```python
from build123d import *

# Parameters (mm, degrees)
F1_DEPTH = 0.25


with BuildPart() as f1:
    # F0 (on Top) → F1 (new body)
    with BuildSketch(Plane.XY):
        with BuildLine():
            ThreePointArc((-0.5, -73.9983107915), (-52.3259018078, -52.3259018078), (-73.9983107915, -0.5))
            Line((-73.9983107915, -0.5), (-49.9974999375, -0.5))
            Line((-49.9974999375, -0.5), (-48.9974489132, -0.5))
            ThreePointArc((-48.9974489132, -0.5), (-49, 0), (-48.9974489132, 0.5))
            ThreePointArc((-48.9974489132, 0.5), (-34.6482322781, 34.6482322781), (-0.5, 48.9974489132))
            Line((-0.5, 48.9974489132), (-0.5, 49.9974999375))
            ThreePointArc((-0.5, 49.9974999375), (-35.3553390593, 35.3553390593), (-49.9974999375, 0.5))
            Line((-49.9974999375, 0.5), (-73.9983107915, 0.5))
            ThreePointArc((-73.9983107915, 0.5), (-52.3259018078, 52.3259018078), (-0.5, 73.9983107915))
            Line((-0.5, 73.9983107915), (-0.5, 74.9983333148))
            ThreePointArc((-0.5, 74.9983333148), (-53.033008589, 53.033008589), (-74.9983333148, 0.5))
            Line((-74.9983333148, 0.5), (-74.9983333148, -0.5))
            ThreePointArc((-74.9983333148, -0.5), (-53.033008589, -53.033008589), (-0.5, -74.9983333148))
            Line((-0.5, -74.9983333148), (-0.5, -73.9983107915))
        make_face()
        with BuildLine():
            Line((-0.5, -49.9974999375), (-0.5, -73.9983107915))
            ThreePointArc((-0.5, -73.9983107915), (0, -74), (0.5, -73.9983107915))
            Line((0.5, -73.9983107915), (0.5, -49.9974999375))
            ThreePointArc((0.5, -49.9974999375), (0, -50), (-0.5, -49.9974999375))
        make_face()
        with BuildLine():
            ThreePointArc((0.5, -73.9983107915), (0, -74), (-0.5, -73.9983107915))
            Line((-0.5, -73.9983107915), (-0.5, -74.9983333148))
            Line((-0.5, -74.9983333148), (0.5, -74.9983333148))
            Line((0.5, -74.9983333148), (0.5, -73.9983107915))
        make_face()
        with BuildLine():
            Line((-48.9974489132, -0.5), (-49.9974999375, -0.5))
            ThreePointArc((-49.9974999375, -0.5), (-35.3553390593, -35.3553390593), (-0.5, -49.9974999375))
            ThreePointArc((-0.5, -49.9974999375), (0, -50), (0.5, -49.9974999375))
            Line((0.5, -49.9974999375), (0.5, -48.9974489132))
            ThreePointArc((0.5, -48.9974489132), (0, -49), (-0.5, -48.9974489132))
            ThreePointArc((-0.5, -48.9974489132), (-34.6482322781, -34.6482322781), (-48.9974489132, -0.5))
        make_face()
        with BuildLine():
            ThreePointArc((73.9983107915, -0.5), (52.3259018078, -52.3259018078), (0.5, -73.9983107915))
            Line((0.5, -73.9983107915), (0.5, -74.9983333148))
            ThreePointArc((0.5, -74.9983333148), (53.033008589, -53.033008589), (74.9983333148, -0.5))
            Line((74.9983333148, -0.5), (73.9983107915, -0.5))
        make_face()
        with BuildLine():
            ThreePointArc((-48.9974489132, 0.5), (-49, 0), (-48.9974489132, -0.5))
            Line((-48.9974489132, -0.5), (-24.9949994999, -0.5))
            Line((-24.9949994999, -0.5), (-23.9947911014, -0.5))
            ThreePointArc((-23.9947911014, -0.5), (-24, 0), (-23.9947911014, 0.5))
            ThreePointArc((-23.9947911014, 0.5), (-16.9705627485, 16.9705627485), (-0.5, 23.9947911014))
            Line((-0.5, 23.9947911014), (-0.5, 24.9949994999))
            ThreePointArc((-0.5, 24.9949994999), (-17.6776695297, 17.6776695297), (-24.9949994999, 0.5))
            Line((-24.9949994999, 0.5), (-48.9974489132, 0.5))
        make_face()
        with BuildLine():
            Line((49.9974999375, -0.5), (73.9983107915, -0.5))
            ThreePointArc((73.9983107915, -0.5), (74, 0), (73.9983107915, 0.5))
            Line((73.9983107915, 0.5), (49.9974999375, 0.5))
            ThreePointArc((49.9974999375, 0.5), (50, 0), (49.9974999375, -0.5))
        make_face()
        with BuildLine():
            ThreePointArc((73.9983107915, 0.5), (74, 0), (73.9983107915, -0.5))
            Line((73.9983107915, -0.5), (74.9983333148, -0.5))
            Line((74.9983333148, -0.5), (74.9983333148, 0.5))
            Line((74.9983333148, 0.5), (73.9983107915, 0.5))
        make_face()
        with BuildLine():
            Line((0.5, -48.9974489132), (0.5, -49.9974999375))
            ThreePointArc((0.5, -49.9974999375), (35.3553390593, -35.3553390593), (49.9974999375, -0.5))
            Line((49.9974999375, -0.5), (48.9974489132, -0.5))
            ThreePointArc((48.9974489132, -0.5), (34.6482322781, -34.6482322781), (0.5, -48.9974489132))
        make_face()
        with BuildLine():
            ThreePointArc((-74.9983333148, 0.5), (-75, 0), (-74.9983333148, -0.5))
            Line((-74.9983333148, -0.5), (-74.9983333148, 0.5))
        make_face()
        with BuildLine():
            Line((-23.9947911014, -0.5), (-24.9949994999, -0.5))
            ThreePointArc((-24.9949994999, -0.5), (-17.6776695297, -17.6776695297), (-0.5, -24.9949994999))
            Line((-0.5, -24.9949994999), (-0.5, -48.9974489132))
            ThreePointArc((-0.5, -48.9974489132), (0, -49), (0.5, -48.9974489132))
            Line((0.5, -48.9974489132), (0.5, -24.9949994999))
            Line((0.5, -24.9949994999), (0.5, -23.9947911014))
            Line((0.5, -23.9947911014), (0.5, -2.4494897428))
            Line((0.5, -2.4494897428), (0.5, -0.5))
            Line((0.5, -0.5), (2.4494897428, -0.5))
            Line((2.4494897428, -0.5), (23.9947911014, -0.5))
            Line((23.9947911014, -0.5), (24.9949994999, -0.5))
            ThreePointArc((24.9949994999, -0.5), (25, 0), (24.9949994999, 0.5))
            Line((24.9949994999, 0.5), (23.9947911014, 0.5))
            Line((23.9947911014, 0.5), (2.4494897428, 0.5))
            Line((2.4494897428, 0.5), (0.5, 0.5))
            Line((0.5, 0.5), (-0.5, 0.5))
            Line((-0.5, 0.5), (-0.5, -0.5))
            Line((-0.5, -0.5), (-0.5, -2.4494897428))
            Line((-0.5, -2.4494897428), (-0.5, -23.9947911014))
            ThreePointArc((-0.5, -23.9947911014), (-16.9705627485, -16.9705627485), (-23.9947911014, -0.5))
        make_face()
        with BuildLine():
            ThreePointArc((0.5, 73.9983107915), (52.3259018078, 52.3259018078), (73.9983107915, 0.5))
            Line((73.9983107915, 0.5), (74.9983333148, 0.5))
            ThreePointArc((74.9983333148, 0.5), (53.033008589, 53.033008589), (0.5, 74.9983333148))
            Line((0.5, 74.9983333148), (0.5, 73.9983107915))
        make_face()
        with BuildLine():
            Line((48.9974489132, -0.5), (49.9974999375, -0.5))
            ThreePointArc((49.9974999375, -0.5), (50, 0), (49.9974999375, 0.5))
            Line((49.9974999375, 0.5), (48.9974489132, 0.5))
            ThreePointArc((48.9974489132, 0.5), (49, 0), (48.9974489132, -0.5))
        make_face()
        with BuildLine():
            Line((-0.5, 49.9974999375), (-0.5, 48.9974489132))
            ThreePointArc((-0.5, 48.9974489132), (0, 49), (0.5, 48.9974489132))
            Line((0.5, 48.9974489132), (0.5, 49.9974999375))
            ThreePointArc((0.5, 49.9974999375), (0, 50), (-0.5, 49.9974999375))
        make_face()
        with BuildLine():
            ThreePointArc((0.5, 48.9974489132), (0, 49), (-0.5, 48.9974489132))
            Line((-0.5, 48.9974489132), (-0.5, 24.9949994999))
            Line((-0.5, 24.9949994999), (-0.5, 23.9947911014))
            ThreePointArc((-0.5, 23.9947911014), (0, 24), (0.5, 23.9947911014))
            ThreePointArc((0.5, 23.9947911014), (16.9705627485, 16.9705627485), (23.9947911014, 0.5))
            Line((23.9947911014, 0.5), (24.9949994999, 0.5))
            ThreePointArc((24.9949994999, 0.5), (17.6776695297, 17.6776695297), (0.5, 24.9949994999))
            Line((0.5, 24.9949994999), (0.5, 48.9974489132))
        make_face()
        with BuildLine():
            ThreePointArc((-23.9947911014, 0.5), (-24, 0), (-23.9947911014, -0.5))
            Line((-23.9947911014, -0.5), (-2.4494897428, -0.5))
            Line((-2.4494897428, -0.5), (-0.5, -0.5))
            Line((-0.5, -0.5), (-0.5, 0.5))
            Line((-0.5, 0.5), (-2.4494897428, 0.5))
            Line((-2.4494897428, 0.5), (-23.9947911014, 0.5))
        make_face()
        with BuildLine():
            Line((0.5, 49.9974999375), (0.5, 73.9983107915))
            ThreePointArc((0.5, 73.9983107915), (0, 74), (-0.5, 73.9983107915))
            Line((-0.5, 73.9983107915), (-0.5, 49.9974999375))
            ThreePointArc((-0.5, 49.9974999375), (0, 50), (0.5, 49.9974999375))
        make_face()
        with BuildLine():
            ThreePointArc((-0.5, 73.9983107915), (0, 74), (0.5, 73.9983107915))
            Line((0.5, 73.9983107915), (0.5, 74.9983333148))
            Line((0.5, 74.9983333148), (-0.5, 74.9983333148))
            Line((-0.5, 74.9983333148), (-0.5, 73.9983107915))
        make_face()
        with BuildLine():
            Line((48.9974489132, 0.5), (49.9974999375, 0.5))
            ThreePointArc((49.9974999375, 0.5), (35.3553390593, 35.3553390593), (0.5, 49.9974999375))
            Line((0.5, 49.9974999375), (0.5, 48.9974489132))
            ThreePointArc((0.5, 48.9974489132), (34.6482322781, 34.6482322781), (48.9974489132, 0.5))
        make_face()
        with BuildLine():
            Line((24.9949994999, -0.5), (48.9974489132, -0.5))
            ThreePointArc((48.9974489132, -0.5), (49, 0), (48.9974489132, 0.5))
            Line((48.9974489132, 0.5), (24.9949994999, 0.5))
            ThreePointArc((24.9949994999, 0.5), (25, 0), (24.9949994999, -0.5))
        make_face()
        with BuildLine():
            Line((0.5, -23.9947911014), (0.5, -24.9949994999))
            ThreePointArc((0.5, -24.9949994999), (17.6776695297, -17.6776695297), (24.9949994999, -0.5))
            Line((24.9949994999, -0.5), (23.9947911014, -0.5))
            ThreePointArc((23.9947911014, -0.5), (16.9705627485, -16.9705627485), (0.5, -23.9947911014))
        make_face()
        with BuildLine():
            ThreePointArc((0.5, 74.9983333148), (0, 75), (-0.5, 74.9983333148))
            Line((-0.5, 74.9983333148), (0.5, 74.9983333148))
        make_face()
        with BuildLine():
            Line((-0.5, -0.5), (-2.4494897428, -0.5))
            ThreePointArc((-2.4494897428, -0.5), (-1.767766953, -1.767766953), (-0.5, -2.4494897428))
            Line((-0.5, -2.4494897428), (-0.5, -0.5))
        make_face()
        with BuildLine():
            ThreePointArc((0.5, 23.9947911014), (0, 24), (-0.5, 23.9947911014))
            Line((-0.5, 23.9947911014), (-0.5, 2.4494897428))
            Line((-0.5, 2.4494897428), (-0.5, 0.5))
            Line((-0.5, 0.5), (0.5, 0.5))
            Line((0.5, 0.5), (0.5, 2.4494897428))
            Line((0.5, 2.4494897428), (0.5, 23.9947911014))
        make_face()
        with BuildLine():
            ThreePointArc((-0.5, 2.4494897428), (-1.767766953, 1.767766953), (-2.4494897428, 0.5))
            Line((-2.4494897428, 0.5), (-0.5, 0.5))
            Line((-0.5, 0.5), (-0.5, 2.4494897428))
        make_face()
        with BuildLine():
            Line((0.5, -0.5), (0.5, -2.4494897428))
            ThreePointArc((0.5, -2.4494897428), (1.767766953, -1.767766953), (2.4494897428, -0.5))
            Line((2.4494897428, -0.5), (0.5, -0.5))
        make_face()
        with BuildLine():
            ThreePointArc((2.4494897428, 0.5), (1.767766953, 1.767766953), (0.5, 2.4494897428))
            Line((0.5, 2.4494897428), (0.5, 0.5))
            Line((0.5, 0.5), (2.4494897428, 0.5))
        make_face()
    extrude(amount=F1_DEPTH)


solid = f1.part
```
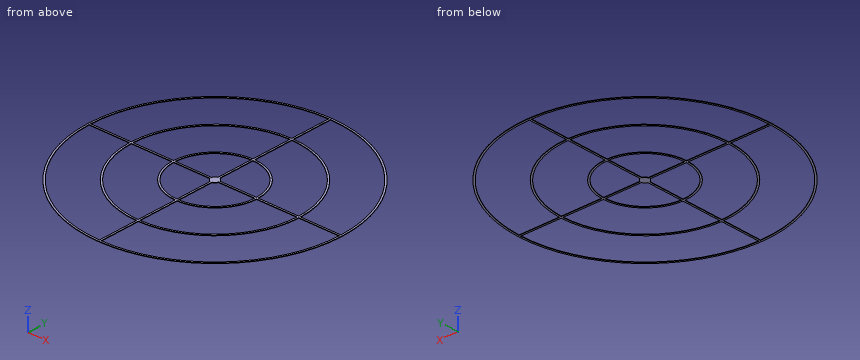
Verification items for the finished model (mm, model axes). Give positions to 0.01 mm unless a question says otherwise; leave off trailing zeros. Loops run counter-clockwise (first coordinate to the right, second up) from the corner with the lowest first, then second, coordinate; pieces in that order, holes last. Notation, with made-up numbers: M -33.5,-12.5 L -17.5,-12.5 A24 cw -17.5,20.5 Z; hole C 38.5,73.25 d4. An arc over 180 degrees is marked long. Return JSON: item names as keys, results as strings.
1) Section check A-A, the plane y = -35.5. Enter the section's corners in (x, z) (3 decimals), and give its area (3 significant figures).
Findings:
{"outline": "M -66.066,0 L -64.929,0 L -64.929,0.25 L -66.066,0.25 Z; M -35.21,0 L -33.775,0 L -33.775,0.25 L -35.21,0.25 Z; M -0.5,0 L 0.5,0 L 0.5,0.25 L -0.5,0.25 Z; M 33.775,0 L 35.21,0 L 35.21,0.25 L 33.775,0.25 Z; M 64.929,0 L 66.066,0 L 66.066,0.25 L 64.929,0.25 Z", "area": "1.54 mm2"}
2) Section check D-D, the plane x = -9.5. Enter the section's corners in (y, z).
Findings:
{"outline": "M -74.4,0 L -73.39,0 L -73.39,0.25 L -74.4,0.25 Z; M -49.09,0 L -48.07,0 L -48.07,0.25 L -49.09,0.25 Z; M -23.12,0 L -22.04,0 L -22.04,0.25 L -23.12,0.25 Z; M -0.5,0 L 0.5,0 L 0.5,0.25 L -0.5,0.25 Z; M 22.04,0 L 23.12,0 L 23.12,0.25 L 22.04,0.25 Z; M 48.07,0 L 49.09,0 L 49.09,0.25 L 48.07,0.25 Z; M 73.39,0 L 74.4,0 L 74.4,0.25 L 73.39,0.25 Z"}
3) Section check B-B, the plane x = -39.5. Enter the section's corners in (y, z).
Findings:
{"outline": "M -63.76,0 L -62.58,0 L -62.58,0.25 L -63.76,0.25 Z; M -30.66,0 L -29,0 L -29,0.25 L -30.66,0.25 Z; M -0.5,0 L 0.5,0 L 0.5,0.25 L -0.5,0.25 Z; M 29,0 L 30.66,0 L 30.66,0.25 L 29,0.25 Z; M 62.58,0 L 63.76,0 L 63.76,0.25 L 62.58,0.25 Z"}
4) Material ranges on L1, parallel to Y at x = -66, z = 0.1; L2, parallel to X at y = 28, z = 0.15; L3, parallel to X at y = 45, z = 0.15, recorded low to high. Write a range as [from, to].
Findings:
{"L1": "y = [-35.62, -33.47], [-0.5, 0.5], [33.47, 35.62]", "L2": "x = [-69.58, -68.5], [-41.42, -40.21], [-0.5, 0.5], [40.21, 41.42], [68.5, 69.58]", "L3": "x = [-60, -58.75], [-21.79, -19.39], [-0.5, 0.5], [19.39, 21.79], [58.75, 60]"}
5) Section check C-C, the plane y = -6. Enter the section's corners in (x, z), and give its area (3 significant figures).
Findings:
{"outline": "M -74.76,0 L -73.76,0 L -73.76,0.25 L -74.76,0.25 Z; M -49.64,0 L -48.63,0 L -48.63,0.25 L -49.64,0.25 Z; M -24.27,0 L -23.24,0 L -23.24,0.25 L -24.27,0.25 Z; M -0.5,0 L 0.5,0 L 0.5,0.25 L -0.5,0.25 Z; M 23.24,0 L 24.27,0 L 24.27,0.25 L 23.24,0.25 Z; M 48.63,0 L 49.64,0 L 49.64,0.25 L 48.63,0.25 Z; M 73.76,0 L 74.76,0 L 74.76,0.25 L 73.76,0.25 Z", "area": "1.77 mm2"}
